Geometry check sheet. Reference: drawing and pictorial views, mm from the part's lowest x, y, z. A direction names the side the tool comes from. Give positions to 0.01 mm unless a question says otherwise; leave off trailing zeros. Order: outer loops, then holes, each group sorted by start corner. A loop starts at its lowest first (then second) coordinate and runs counter-clockwise, first axis right, second up.
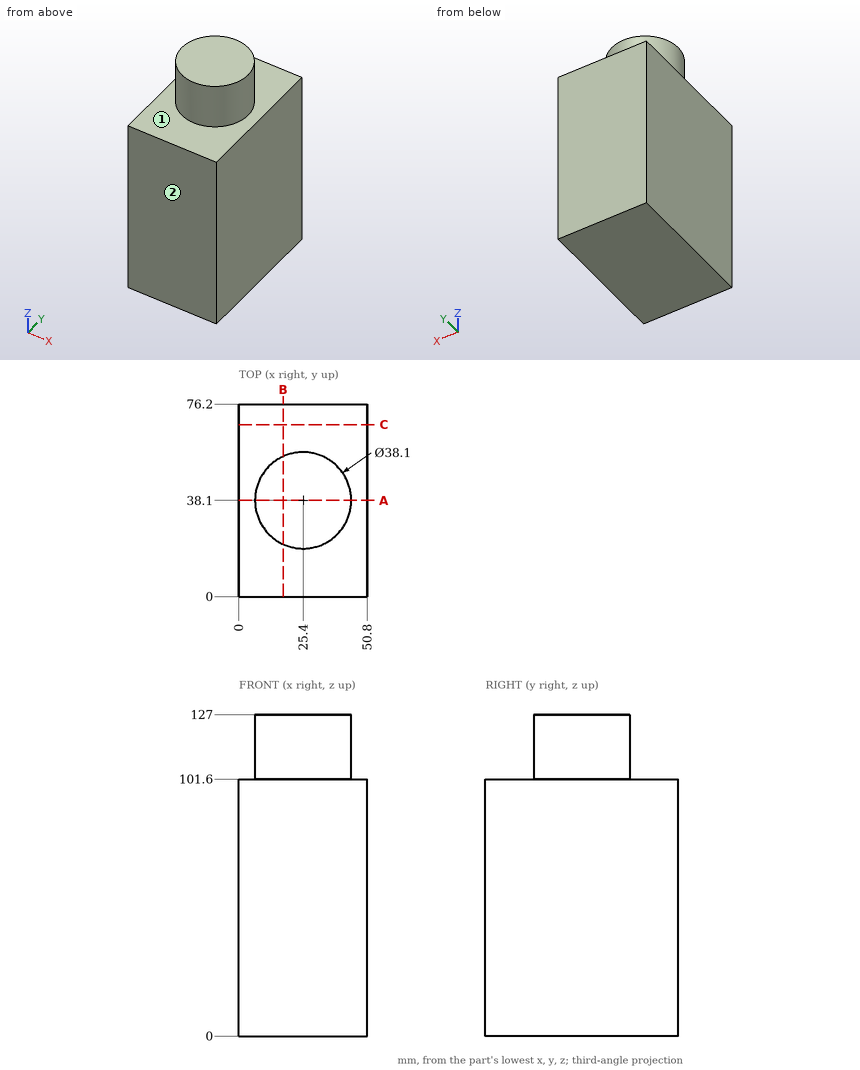
(1) Cross-section at A-A on y = 38.1. Enter the section's corners in (x, z).
Response values:
outline: (0, 0) - (50.8, 0) - (50.8, 101.6) - (44.45, 101.6) - (44.45, 127) - (6.35, 127) - (6.35, 101.6) - (0, 101.6) - close
(2) Material ranges on L1, parallel to Z at x = 31.5, y = 11; L2, parallel to X at y = 37.5, z = 117; L3, parallel to X at y = 29.5, z = 108, recorded low to high.
Response values:
L1: z = 0 to 101.6
L2: x = 6.36 to 44.44
L3: x = 8.4 to 42.4
(3) Gauge pin test, flat ends, axial feed: pin 1 Ø1.5 at (x, y) = (41.5, 59.5) entering from -Z; pin 2 Ø4 at (y, z) = (17, 109.5) entering from +X; pin 3 Ø2 at (x, z) = (20.5, 112) entering from +Y. Record the tip position at first contact, or that the pin passes through.
Response values:
pin 1: stops at z = 0
pin 2: passes through
pin 3: stops at y = 56.75
(4) Set-up check for the marked faces 1 and 2: record each of +Z, -Z, +X, -X, +Y, -Y from which the full face is reachable in a straight line by a thin tool's end or side.
Response values:
face 1: +Z
face 2: +Z, -Z, +X, -X, -Y
(5) Cross-section at B-B on x = 17.5. Enter the section's corners in (y, z), then the cut area to 3 significant figures.
Response values:
outline: (0, 0) - (76.2, 0) - (76.2, 101.6) - (55.43, 101.6) - (55.43, 127) - (20.77, 127) - (20.77, 101.6) - (0, 101.6) - close
area: 8,620 mm2
(6) Cross-section at C-C on y = 68. Enter the section's corners in (x, z).
Response values:
outline: (0, 0) - (50.8, 0) - (50.8, 101.6) - (0, 101.6) - close
